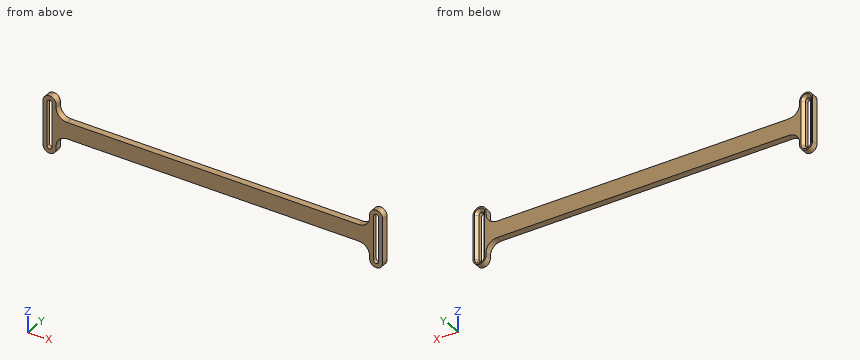
from build123d import *

# Parameters (mm, degrees)
BOSS_EXTRUDE1_DEPTH = 6
FILLET1_R           = 10
FILLET2_R           = 2.25
FILLET3_R           = 6
CHAMFER1_SIZE       = 2.5


with BuildPart() as part:
    # Sketch1 → Boss-Extrude1 (new body)
    with BuildSketch(Plane(origin=(0, 0, 0), x_dir=(1, 0, 0), z_dir=(0, 1, 0))):
        Polygon((-152.25, 0), (-156, 0), (-156, -26), (-144, -26), (-144, -7.5), (0, -7.5), (0, 0), (-85.684931507, 0), (-147.75, 0), (-147.75, -22.25), (-152.25, -22.25), align=None)
    extrude(amount=BOSS_EXTRUDE1_DEPTH)

    # Fillet1
    fillet1_edges = [part.edges().sort_by_distance(p)[0] for p in [
        (-144, 3, 7.5),
    ]]
    fillet(fillet1_edges, radius=FILLET1_R)

    # Fillet2
    fillet2_edges = [part.edges().sort_by_distance(p)[0] for p in [
        (-152.25, 3, 22.25),
        (-147.75, 3, 22.25),
    ]]
    fillet(fillet2_edges, radius=FILLET2_R - 0.0001)  # a hair under: the kernel refuses the full size

    # Fillet3
    fillet3_edges = [part.edges().sort_by_distance(p)[0] for p in [
        (-156, 3, 26),
        (-144, 3, 26),
    ]]
    fillet(fillet3_edges, radius=FILLET3_R - 0.0001)  # a hair under: the kernel refuses the full size

    # Chamfer1
    chamfer1_edges = [part.edges().sort_by_distance(p)[0] for p in [
        (-152.25, 6, 10.00005),
        (-147.75, 6, 10.00005),
        (-151.591019547, 6, 21.591019547),
        (-148.408980453, 6, 21.591019547),
    ]]
    chamfer(chamfer1_edges, length=CHAMFER1_SIZE)

    # Mirror1: part across plane


with BuildPart() as part_1:
    add(part.part)
    add(part.part.mirror(Plane(origin=(0, 6, 0), x_dir=(1, 0, 0), z_dir=(0, 0, 1))))

    # Mirror2: part across plane


with BuildPart() as part_2:
    add(part_1.part)
    add(part_1.part.mirror(Plane(origin=(0, 6, 0), x_dir=(0, 0, 1), z_dir=(1, 0, 0))))


solid = part_2.part
For this review, take the finished solid that the model builds, in its own axes (mm). Give positions to 0.01 mm unless a question says otherwise; leave off trailing zeros. Order: outer loops, then holes, each group sorted by start corner. A loop starts at its lowest first (then second) coordinate and runs counter-clockwise, first axis right, second up. Notation, with made-up numbers: (-32, 82) - (0, 82) arc R19 cw to (0, 93) - close; hole circle Ø9 at (-15.5, -35). An arc over 180 degrees is marked (long way). Answer as a JSON object with one key per item and string values. Group by question number.
Item 1: Take a section at B-B on y = 5. Give the number of separate pieces and of enclosed holes in the cut face, and give its area (3 significant figures).
Item 2: Take a section at A-A on z = -4. Give the boundary of the cut face in (x, y).
Item 3: Take a section at C-C on x = -58. Give the boundary of the cut face in (y, z).
Item 4: Wall thickness on line 1 along X through (y, z) = (3.25, -17.5); line 2 along X through (y, z) = (1.75, -6); line 3 along X through (y, z) = (4.5, -12.5): over which ranges is each line inside the solid? List them lowest first.
Item 5: Clearance check with flat-ended pins moving along their axes: pin 1 Ø12 at (x, z) = (-1, 10.5) entering from +Y; pin 2 Ø3 at (x, y) = (-40, 4.5) entering from -Z; pin 3 Ø1.8 at (x, y) = (21, 2) entering from +Z. State where each tip first meets the part, or that it passes through.
Reported:
{
 "1": {"separate pieces": "1", "enclosed holes": "2", "area": "4,900 mm^2"},
 "2": {"outline": "(-156, 0) - (-152.25, 0) - (-152.25, 3.5) - (-154.75, 6) - (-156, 6) - close; (-147.75, 0) - (147.75, 0) - (147.75, 3.5) - (145.25, 6) - (-145.25, 6) - (-147.75, 3.5) - close; (152.25, 0) - (156, 0) - (156, 6) - (154.75, 6) - (152.25, 3.5) - close"},
 "3": {"outline": "(0, -7.5) - (6, -7.5) - (6, 7.5) - (0, 7.5) - close"},
 "4": {"line 1": "-156 to -152.25, -147.75 to -144, 144 to 147.75, 152.25 to 156", "line 2": "-156 to -152.25, -147.75 to 147.75, 152.25 to 156", "line 3": "-156 to -153.25, -146.75 to -142.66, 142.66 to 146.75, 153.25 to 156"},
 "5": {"pin 1": "y = 6", "pin 2": "z = -7.5", "pin 3": "z = 7.5"}
}
